Geometry check sheet. Reference: the model listing, model coordinates, mm. Give positions to 0.01 mm unless a question says otherwise; leave off trailing zeros. Write each loop counter-clockwise with the first axis right and the second up, starting at its lowest first coordinate (ties: lowest second). Pieces come first, ordered by that corner, then holes.
(1) Mould release check, pull along X, two halves, no side actions. Record for faces 1 (the cylindrical face through (-14.874, -5.91, -26.06)), 2 (the flat face through (92.889, -6, 1)), 3 (the cylindrical face through (-12.683, -5.91, 35.454)), 4 (the flat face through (19, -6, 39.31)): +X half, -X half, draft (parallel to the pull), parting line (faces both ways), or undercut.
(2) Thickness scan on line 1 along Z through (x, y) = (3, -1.75); line 2 along Z through (x, y) = (82, -4); line 3 along X through (y, z) = (-8.5, -23). Record the ranges inside material, lowest first.
(3) Cross-section at A-A (x = 3.5). Record the boundary of the cut face in (y, z).
(4) Cross-section at B-B (y = -8.25). Count the separate pieces of the cut face and the enclosed holes in it, and give its area (3 significant figures).
```python
from build123d import *

# Parameters (mm, degrees)
F0_R     = 3.302051
F0_R_2   = 3.302054
F0_R_3   = 3.378854
F0_R_4   = 3.203462
F0_R_5   = 3.397783
F1_DEPTH = 11.9888


with BuildPart() as f1:
    # F0 (on Front) → F1 (new body)
    with BuildSketch(Plane.XZ):
        Polygon((92.889122, 39.310039), (-57.123278, 39.310039), (-57.123278, -31.973779), (-57.123278, -36.686761), (92.889122, -36.686761), align=None)
        with Locations((-44.845879, -24.050448)):
            Circle(F0_R, mode=Mode.SUBTRACT)
        with Locations((-29.44508, -24.050448)):
            Circle(F0_R, mode=Mode.SUBTRACT)
        with Locations((-12.253493, -24.050448)):
            Circle(F0_R, mode=Mode.SUBTRACT)
        with Locations((3.86362, -24.050448)):
            Circle(F0_R, mode=Mode.SUBTRACT)
        with Locations((-44.845879, 32.180369)):
            Circle(F0_R, mode=Mode.SUBTRACT)
        with Locations((-29.44508, 32.180369)):
            Circle(F0_R_2, mode=Mode.SUBTRACT)
        with Locations((-12.253493, 32.180369)):
            Circle(F0_R, mode=Mode.SUBTRACT)
        with Locations((3.86362, 32.180369)):
            Circle(F0_R, mode=Mode.SUBTRACT)
        with Locations((62.959701, 22.5101)):
            Circle(F0_R_3, mode=Mode.SUBTRACT)
        with Locations((83.374709, 22.5101)):
            Circle(F0_R_4, mode=Mode.SUBTRACT)
        with Locations((62.959701, 32.180369)):
            Circle(F0_R_5, mode=Mode.SUBTRACT)
        with Locations((83.374709, 32.180369)):
            Circle(F0_R_5, mode=Mode.SUBTRACT)
    extrude(amount=F1_DEPTH)


solid = f1.part
```
Reply:
1. face 1: undercut
1. face 2: +X half
1. face 3: undercut
1. face 4: draft
2. line 1: z = -36.69 to -27.24, -20.86 to 28.99, 35.37 to 39.31
2. line 2: z = -36.69 to 19.62, 25.4 to 29.07, 35.29 to 39.31
2. line 3: x = -57.12 to -47.98, -41.72 to -32.58, -26.31 to -15.38, -9.12 to 0.73, 6.99 to 92.89
3. outline: (-11.99, -36.69) - (0, -36.69) - (0, -27.33) - (-11.99, -27.33) - close; (-11.99, -20.77) - (0, -20.77) - (0, 28.9) - (-11.99, 28.9) - close; (-11.99, 35.46) - (0, 35.46) - (0, 39.31) - (-11.99, 39.31) - close
4. separate pieces: 1
4. enclosed holes: 12
4. area: 11,000 mm2
